Can you work these out from the model? Positions are in its coordinate system, mm. A direction names the side the tool comes from. Coordinates: 2 decimals unless noted, no trailing zeros. Order: outer loops, then holes, each group sorted by start corner. A loop starts at its lowest first (then second) coordinate and runs counter-clockwise, first axis right, second up. Notation, with made-up numbers: (-21, 0) -> (9, 0) arc R24 cw to (9, 10) -> close; hole circle Ø5 at (61.25, 23). An arc over 180 degrees is marked (long way). Answer in a Markdown table with one row per item. Add a question column.
1. Imagine slicing it at C-C on x = -63.5. Write out the boundary of the cut face in (y, z), plus the area to 3 significant figures.
2. On a 3-axis mill with a long thin cutter (end or side, diameter ignored), from which of +Z, -Z, +X, -X, +Y, -Y can I reach the whole of each face in a straight line? I mean faces 4 (the face through (22.264, 14.039, 1.252)), 5 (the face through (3, 2.54, 8)). Say none if no direction works.
3. We'd pull the mould along Z, two halves only. Please class faces 1 (the face through (37.4, 12.8, 1.3)), 2 (the face through (3, 13, 0)), 3 (the face through (-75.896, 24.112, 6.42)): pulls with the +Z half, pulls with the -Z half, needs draft (parallel to the pull), parting line crosses it, or undercut.
4. Imagine slicing it at A-A on z = 6.35. Write out the boundary of the cut face in (x, y).
5. Will this pin go through, and if not, where does the flat tip stop? pin 1 (3.5 mm diameter, centred on x = 23.12, y = 12.7, fed in from +Z).
6. Imagine slicing it at B-B on y = 12.7. Write out the boundary of the cut face in (x, z).
7. Imagine slicing it at D-D on y = 20.75. Write out the boundary of the cut face in (x, z), plus the area to 3 significant figures.
8. If I drill on line 1 along X through (y, z) = (1.5, 6); line 2 along Y through (x, z) = (21, 8.25); line 3 along Z through (x, y) = (-52.5, 15.25), over which ranges is the centre line in solid material (lowest first)? Write a range as [from, to].
from build123d import *

# Parameters (mm, degrees)
F0_W     = 190.5
F0_H     = 25.4
F1_DEPTH = 12.7
F2_T     = -2.54
F4_D     = 3.175
F6_D     = 3.175


with BuildPart() as f1:
    # F0 (on Top) → F1 (new body)
    with BuildSketch(Plane.XY):
        with Locations((4.067147, 12.7)):
            Rectangle(F0_W, F0_H)
    extrude(amount=F1_DEPTH)

    # F2
    f2_openings = [f1.faces().sort_by_distance(p)[0] for p in [
        (4.067147, 12.7, 12.7),
        (99.317147, 12.7, 6.35),
        (-91.182853, 12.7, 6.35),
    ]]
    offset(amount=F2_T, openings=f2_openings)

    # F4 (through all)
    with Locations(Plane.XY.offset(2.54)):
        with Locations((10.417147, 12.7), (23.117147, 12.7), (35.817147, 12.7), (86.617147, 12.7)):
            Hole(F4_D / 2)

    # F6 (through all)
    with Locations(Plane(origin=(0, 25.4, 0), x_dir=(-1, 0, 0), z_dir=(0, 1, 0))):
        with Locations((74.310439, 6.35), (82.716187, 6.35)):
            Hole(F6_D / 2)


solid = f1.part
Answers follow:
| question | item | result |
|---|---|---|
| 1 | outline | (0, 0) -> (25.4, 0) -> (25.4, 12.7) -> (22.86, 12.7) -> (22.86, 2.54) -> (2.54, 2.54) -> (2.54, 12.7) -> (0, 12.7) -> close |
| 1 | area | 116 mm² |
| 2 | face 4 | +Z, -Z |
| 2 | face 5 | +Z, +X, -X |
| 3 | face 1 | needs draft |
| 3 | face 2 | pulls with the -Z half |
| 3 | face 3 | undercut |
| 4 | outline | (-91.18, 0) -> (-84.3, 0) -> (-84.3, 2.54) -> (-91.18, 2.54) -> close; (-91.18, 22.86) -> (-84.3, 22.86) -> (-84.3, 25.4) -> (-91.18, 25.4) -> close; (-81.13, 0) -> (-75.9, 0) -> (-75.9, 2.54) -> (-81.13, 2.54) -> close; (-81.13, 22.86) -> (-75.9, 22.86) -> (-75.9, 25.4) -> (-81.13, 25.4) -> close; (-72.72, 0) -> (99.32, 0) -> (99.32, 2.54) -> (-72.72, 2.54) -> close; (-72.72, 22.86) -> (99.32, 22.86) -> (99.32, 25.4) -> (-72.72, 25.4) -> close |
| 5 | pin 1 | stops at z = 2.54 |
| 6 | outline | (-91.18, 0) -> (8.83, 0) -> (8.83, 2.54) -> (-91.18, 2.54) -> close; (12, 0) -> (21.53, 0) -> (21.53, 2.54) -> (12, 2.54) -> close; (24.7, 0) -> (34.23, 0) -> (34.23, 2.54) -> (24.7, 2.54) -> close; (37.4, 0) -> (85.03, 0) -> (85.03, 2.54) -> (37.4, 2.54) -> close; (88.2, 0) -> (99.32, 0) -> (99.32, 2.54) -> (88.2, 2.54) -> close |
| 7 | outline | (-91.18, 0) -> (99.32, 0) -> (99.32, 2.54) -> (-91.18, 2.54) -> close |
| 7 | area | 484 mm² |
| 8 | line 1 | x = [-91.18, -84.26], [-81.17, -75.86], [-72.76, 99.32] |
| 8 | line 2 | y = [0, 2.54], [22.86, 25.4] |
| 8 | line 3 | z = [0, 2.54] |
